```python
from build123d import *

# Parameters (mm, degrees)
BOSS_EXTRUDE1_DEPTH     = 40
SKETCH2_R               = 1.5
CUT_EXTRUDE1_DEPTH      = 3
SKETCH3_W               = 15
SKETCH3_H               = 10
CUT_EXTRUDE_THIN1_DEPTH = 46.956501172


with BuildPart() as part:
    # Sketch1 → Boss-Extrude1 (new body)
    with BuildSketch(Plane.XY):
        with BuildLine():
            Line((-2.633913438, -13.75), (-16, -13.75))
            Line((-16, -13.75), (-16, 0))
            ThreePointArc((-16, 0), (0, 16), (16, 0))
            Line((16, 0), (16, -13.75))
            Line((16, -13.75), (2.633913438, -13.75))
            ThreePointArc((2.633913438, -13.75), (0, 14), (-2.633913438, -13.75))
        make_face()
    extrude(amount=BOSS_EXTRUDE1_DEPTH)

    # Sketch2 → Cut-Extrude1 (cut)
    with BuildSketch(Plane.XZ.offset(13.75)):
        with Locations((13, 33.333333333)):
            Circle(SKETCH2_R)
        with Locations((13, 20)):
            Circle(SKETCH2_R)
        with Locations((13, 6.666666667)):
            Circle(SKETCH2_R)
        with Locations(Location((-13, 6.666666667, 0), (0, 0, 180))):
            Circle(SKETCH2_R)
        with Locations(Location((-13, 20, 0), (0, 0, 180))):
            Circle(SKETCH2_R)
        with Locations(Location((-13, 33.333333333, 0), (0, 0, 180))):
            Circle(SKETCH2_R)
    extrude(amount=-CUT_EXTRUDE1_DEPTH, mode=Mode.SUBTRACT)

    # Sketch3 → Cut-Extrude-Thin1 (cut, through all)
    with BuildSketch(Plane.XY.offset(40)):
        with Locations((0, -8.75)):
            Rectangle(SKETCH3_W, SKETCH3_H)
    extrude(amount=-CUT_EXTRUDE_THIN1_DEPTH, mode=Mode.SUBTRACT)


solid = part.part
```
The model under review builds one solid part; all positions refer to its coordinate system, in mm. A direction names the side the tool comes from. Round coordinates to 2 decimals unless told otherwise and drop trailing zeros. Order: outer loops, then holes, each group sorted by start corner. A loop starts at its lowest first (then second) coordinate and runs counter-clockwise, first axis right, second up. Notation, with made-up numbers: (59.5, 48.5) -> (83.5, 48.5) arc R27 ccw to (83.5, 87.5) -> close; hole circle Ø10 at (0.25, 57.5). An arc over 180 degrees is marked (long way). Use a Markdown table: item, result.
Q1. Mouldability with a two-part tool opening along X and no side actions: class faces 4 (the flat face through (-16, -7, 20)), 5 (the cylindrical face through (-11.89, -12.27, 18.99)), 6 (the cylindrical face through (11.5, -12.3, 6.7)), 7 (the flat face through (-11, -13.75, 20)) as +X half, -X half, draft (parallel to the pull), parting line (faces both ways), or undercut.
Values:
| item | result |
|---|---|
| face 4 | -X half |
| face 5 | undercut |
| face 6 | undercut |
| face 7 | draft |
Q2. For line 1 (Z direction, x = -13, y = -12.35); line 2 (X direction, y = 11, z = 12.5); line 3 (X direction, y = 7, z = 13), list the stretches that pass through material, from the lowest coordinate up.
Values:
| item | result |
|---|---|
| line 1 | z = 0 to 5.17, 8.17 to 18.5, 21.5 to 31.83, 34.83 to 40 |
| line 2 | x = -11.62 to -8.66, 8.66 to 11.62 |
| line 3 | x = -14.39 to -12.12, 12.12 to 14.39 |
Q3. We need section A-A on x = -11. Write out the cut boundary in (y, z).
Values:
| item | result |
|---|---|
| outline | (-13.75, 0) -> (-8.66, 0) -> (-8.66, 40) -> (-13.75, 40) -> close; (8.66, 0) -> (11.62, 0) -> (11.62, 40) -> (8.66, 40) -> close |
Q4. We need section D-D on z = 20. Write out the cut boundary in (x, y).
Values:
| item | result |
|---|---|
| outline | (-16, -13.75) -> (-14.5, -13.75) -> (-14.5, -10.75) -> (-11.5, -10.75) -> (-11.5, -13.75) -> (-7.5, -13.75) -> (-7.5, -11.82) arc R14 cw (long way) to (7.5, -11.82) -> (7.5, -13.75) -> (11.5, -13.75) -> (11.5, -10.75) -> (14.5, -10.75) -> (14.5, -13.75) -> (16, -13.75) -> (16, 0) arc R16 ccw to (-16, 0) -> close |
Q5. We need section C-C on y = -0.5. Write out the cut boundary in (x, z), then the cut area to 3 significant figures.
Values:
| item | result |
|---|---|
| outline | (-16, 0) -> (-13.99, 0) -> (-13.99, 40) -> (-16, 40) -> close; (13.99, 0) -> (16, 0) -> (16, 40) -> (13.99, 40) -> close |
| area | 161 mm^2 |
Q6. Tool access review of faces 1 (the flat face through (-7.5, -13, 20)), 2 (the flat face through (12, -8, 0)), 3 (the flat face through (-13, -10.75, 7)): name each direction out of +Z, -Z, +X, -X, +Y, -Y from which nothing blocks a thin tool from reaching the whole face with its end or side.
Values:
| item | result |
|---|---|
| face 1 | +Z, -Z, -Y |
| face 2 | -Z, +X, -X, +Y, -Y |
| face 3 | -Y |
Q7. Clearance check with flat-ended pins moving along their axes: P1, Ø1.5, axis at x = -12.5, z = 7, coming from the -Y side; P2, Ø8, axis at x = -9, z = 27, coming from the +Y side; P3, Ø4, axis at x = -13, z = 33.33, coming from the +Y side. State where each tip first meets the part, or that it passes through.
Values:
| item | result |
|---|---|
| P1 | stops at y = -10.75 |
| P2 | stops at y = 15.2 |
| P3 | stops at y = 11.62 |
Q8. We need section B-B on z = 26. Write out the cut boundary in (x, y).
Values:
| item | result |
|---|---|
| outline | (-16, -13.75) -> (-7.5, -13.75) -> (-7.5, -11.82) arc R14 cw (long way) to (7.5, -11.82) -> (7.5, -13.75) -> (16, -13.75) -> (16, 0) arc R16 ccw to (-16, 0) -> close |
